For this review, use the dimensioned drawing (mm, ordinates from the lowest corner) and the shaded views. A direction names the side the tool comes from. Coordinates: 2 decimals unless noted, no trailing zeros. Loops run counter-clockwise (first coordinate to the right, second up) from the corner with the lowest first, then second, coordinate; pieces in that order, holes last. Notation, with made-up numbers: (6.5, 10) - (47.5, 10) arc R21 cw to (47.5, 40) - close; hole circle Ø10 at (40.25, 80.25). An arc over 180 degrees is marked (long way). Use a Markdown table: item, result. Add a question column.
1) For the marked faces 1 and 2, list the 3-axis set-ups (+Z, -Z, +X, -X, +Y, -Y) from which the entire face can be reached by the end or side of a thin tool; tool diameter is ignored.
2) Add section C-C, the plane z = 2.75. Give the boundary of the cut face in (x, y).
3) To check wall thickness, follow L1, parallel to Y at x = 6, z = 5; L2, parallel to X at y = 7.25, z = 6.5; L3, parallel to Z at x = 3.75, y = 6.5. State the ranges of each line that lie inside material, in increasing order. Write a range as [from, to].
4) Add section D-D, the plane x = 0.75. Give the boundary of the cut face in (y, z).
5) Add section B-B, the plane y = 4. Give the boundary of the cut face in (x, z).
6) Add section A-A, the plane z = 6.25. Give the boundary of the cut face in (x, y), and give its area (3 significant figures).
7) The part is to be moulded in two halves that separate along X. For the marked faces 3, 4 and 5, say which applies: pulls with the +X half, pulls with the -X half, needs draft (parallel to the pull), parting line crosses it, or undercut.
8) Clearance check with a flat-ended pin moving along its axis: pin 1 (1.5 mm diameter, centred on x = 2, y = 3, fed in from +Z). State where the tip first meets the part, or that it passes through.
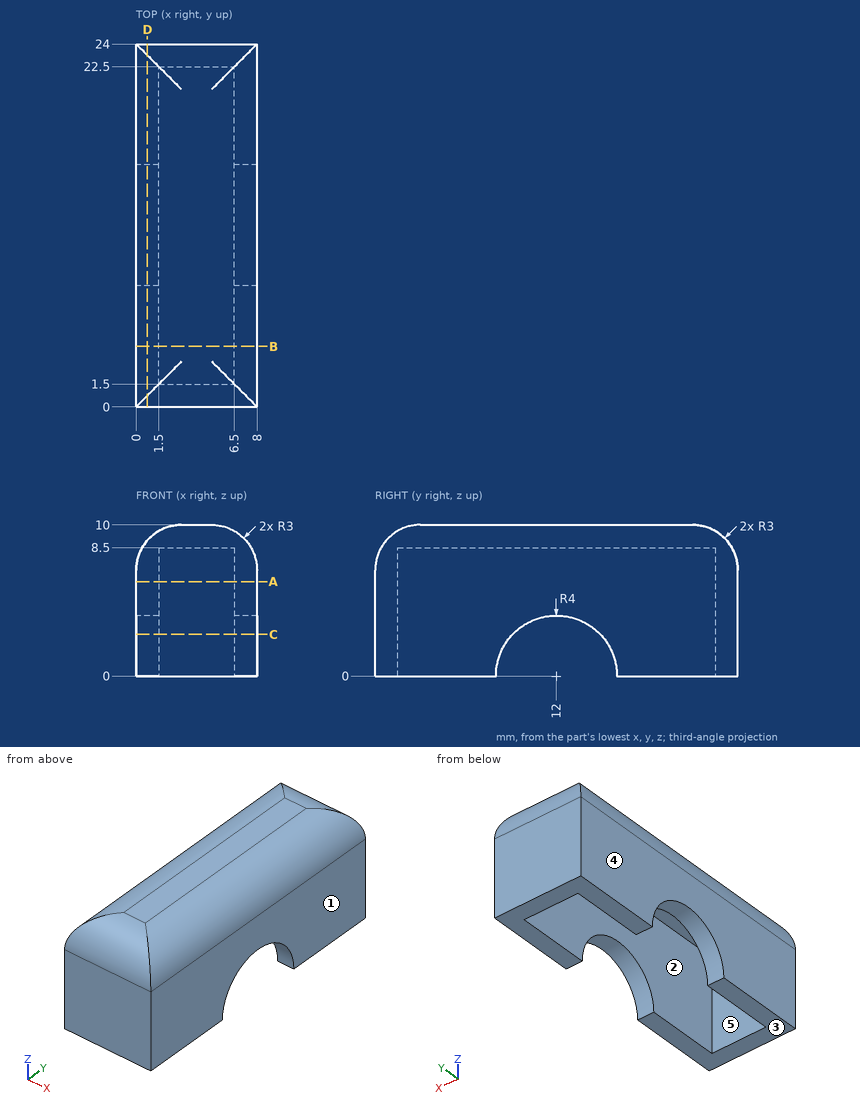
From the geometry:
| question | item | result |
|---|---|---|
| 1 | face 1 | +Z, -Z, +X, +Y, -Y |
| 1 | face 2 | -Z |
| 2 | outline | (0, 0) - (8, 0) - (8, 9.1) - (6.5, 9.1) - (6.5, 1.5) - (1.5, 1.5) - (1.5, 9.1) - (0, 9.1) - close; (0, 14.9) - (1.5, 14.9) - (1.5, 22.5) - (6.5, 22.5) - (6.5, 14.9) - (8, 14.9) - (8, 24) - (0, 24) - close |
| 3 | L1 | y = [0, 1.5], [22.5, 24] |
| 3 | L2 | x = [0, 1.5], [6.5, 8] |
| 3 | L3 | z = [8.5, 10] |
| 4 | outline | (0, 0) - (8, 0) arc R4 cw to (16, 0) - (24, 0) - (24, 7) arc R3 ccw to (23.25, 8.98) - (0.75, 8.98) arc R3 ccw to (0, 7) - close |
| 5 | outline | (0, 0) - (1.5, 0) - (1.5, 8.5) - (6.5, 8.5) - (6.5, 0) - (8, 0) - (8, 7) arc R3 ccw to (5, 10) - (3, 10) arc R3 ccw to (0, 7) - close |
| 6 | outline | (0, 0) - (8, 0) - (8, 24) - (0, 24) - close; hole (1.5, 1.5) - (6.5, 1.5) - (6.5, 22.5) - (1.5, 22.5) - close |
| 6 | area | 87.0 mm^2 |
| 7 | face 3 | needs draft |
| 7 | face 4 | pulls with the -X half |
| 7 | face 5 | undercut |
| 8 | pin 1 | stops at z = 9.99 |
